Design review of the part built by this model. Coordinates are the model's own, in mm. Face numbers are marked on the shaded views. Give positions to 0.01 mm unless a question says otherwise; leave off trailing zeros. Order: outer loops, then holes, each group sorted by start corner. A loop starts at its lowest first (then second) coordinate and runs counter-clockwise, first axis right, second up. Notation, with made-up numbers: M -29,-6.5 L 4,-6.5 A19 cw 4,8.5 Z; hole C 33,27 d10. An arc over 180 degrees is marked long. Answer as a JSON object with one key per item and string values.
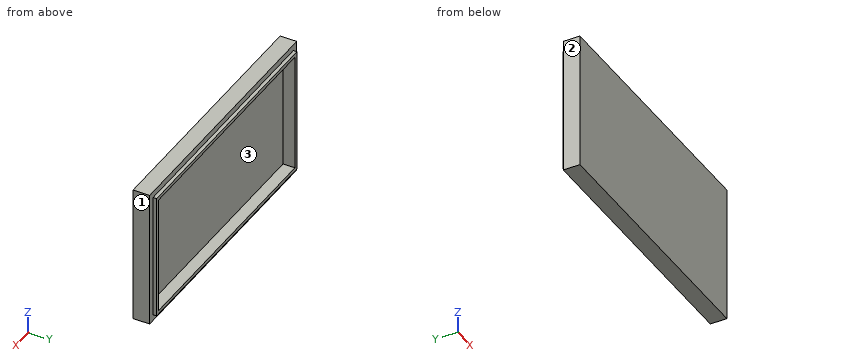
Autodesk Fusion 360 part; units mm, degrees
sketch "Sketch1" plane through (0, 0, 0) normal (0, 1, 0) x (1, 0, 0)
  line L0 (0, 0) -> (95.5, 0)
  line L1 (95.5, 0) -> (95.5, 50)
  line L2 (95.5, 50) -> (0, 50)
  line L3 (0, 50) -> (0, 0)
  dimension "d1" = 95.5
  dimension "d2" = 50
extrude "Extrude1" add sketch "Sketch1" along normal blind 6
sketch "Sketch3" plane through (0, 6, 0) normal (0, 1, 0) x (-1, 0, 0)
  line L0 (0, -50) -> (0, 0)
  line L1 (0, 0) -> (-95.5, 0)
  line L2 (-95.5, 0) -> (-95.5, -50)
  line L3 (-95.5, -50) -> (0, -50)
  line L4 (-2.2, -2.2) -> (-93.3, -2.2)
  line L5 (-93.3, -2.2) -> (-93.3, -47.8)
  line L6 (-93.3, -47.8) -> (-2.2, -47.8)
  line L7 (-2.2, -47.8) -> (-2.2, -2.2)
  dimension "d7" = 91.1
  dimension "d8" = 45.6
extrude "Extrude2" cut sketch "Sketch3" against normal blind 3 contours L4 L5 L6 L7
sketch "Sketch4" plane through (0, 3, 0) normal (0, 1, 0) x (-1, 0, 0)
  line L0 (-2.2, -47.8) -> (-2.2, -2.2)
  line L1 (-2.2, -2.2) -> (-93.3, -2.2)
  line L2 (-93.3, -2.2) -> (-93.3, -47.8)
  line L3 (-93.3, -47.8) -> (-2.2, -47.8)
  line L4 (-3.5, -3.5) -> (-92, -3.5)
  line L5 (-92, -3.5) -> (-92, -46.5)
  line L6 (-92, -46.5) -> (-3.5, -46.5)
  line L7 (-3.5, -46.5) -> (-3.5, -3.5)
  dimension "d11" = 88.5
  dimension "d12" = 43
extrude "Extrude3" add sketch "Sketch4" along normal blind 4.3
(1) Draft analysis for pull direction X (two halves, no side actions). For the marked faces 1, 2 and 3, state which applies: +X half, -X half, draft (parallel to the pull), parting line (faces both ways), or undercut.
Checked values:
{"face 1": "+X half", "face 2": "-X half", "face 3": "undercut"}
(2) We need section A-A (y = 4). Write out the cut boundary in (x, z), plus the area to 4 significant figures.
Checked values:
{"outline": "M 0,-50 L 95.5,-50 L 95.5,0 L 0,0 Z; hole M 3.5,-46.5 L 92,-46.5 L 92,-3.5 L 3.5,-3.5 Z", "area": "969.5 mm^2"}
(3) Insertion check: pin 1 (2 mm diameter, centred on x = 38, z = -30, fed in from -Y); pin 2 (21.5 mm diameter, centred on x = 67, z = -35, fed in from +Y). Each pin has a flat end and moves straight along its axis. Give the tip position at first contact, or say it passes through.
Checked values:
{"pin 1": "stops at y = 0", "pin 2": "stops at y = 3"}
(4) We need section B-B (x = 31). Write out the cut boundary in (y, z).
Checked values:
{"outline": "M 0,-50 L 6,-50 L 6,-47.8 L 7.3,-47.8 L 7.3,-46.5 L 3,-46.5 L 3,-3.5 L 7.3,-3.5 L 7.3,-2.2 L 6,-2.2 L 6,0 L 0,0 Z"}
(5) To check wall thickness, follow L1, parallel to X at y = 5.25, z = -43; L2, parallel to Z at x = 37.5, y = 4.25; L3, parallel to Z at x = 81, y = 7. State the ranges of each line that lie inside material, in increasing order. Write a range as from..to.
Checked values:
{"L1": "x = 0..3.5, 92..95.5", "L2": "z = -50..-46.5, -3.5..0", "L3": "z = -47.8..-46.5, -3.5..-2.2"}
(6) We need section C-C (z = -41). Write out the cut boundary in (x, y).
Checked values:
{"outline": "M 0,0 L 95.5,0 L 95.5,6 L 93.3,6 L 93.3,7.3 L 92,7.3 L 92,3 L 3.5,3 L 3.5,7.3 L 2.2,7.3 L 2.2,6 L 0,6 Z"}
